Geometry: final body of the model. Coordinates: model frame, mm. A direction names the side the tool comes from. Give positions to 0.01 mm unless a question says otherwise; leave off trailing zeros. Write each loop counter-clockwise with the first axis right and the second up, starting at its lowest first coordinate (ties: lowest second). Pieces come first, ordered by that corner, then holes.
```python
from build123d import *

# Parameters (mm, degrees)
F0_W      = 69.85
F0_H      = 69.85
F1_DEPTH  = 1.5875
F2_W      = 69.85
F2_H      = 69.85
F2_W_2    = 66.675
F2_H_2    = 66.675
F3_DEPTH  = 42.8625
F4_W      = 60.325
F4_H      = 60.325
F4_W_2    = 57.15
F4_H_2    = 57.15
F5_DEPTH  = 74.6125
F6_W      = 57.15
F6_H      = 1.5875
F7_DEPTH  = 58.7375
F8_R      = 25.4
F9_DEPTH  = 74.6125
F10_R     = 26.9875
F10_R_2   = 25.4
F11_DEPTH = 76.2


with BuildPart() as f1:
    # F0 (on Top) → F1 (new body)
    with BuildSketch(Plane.XY):
        Rectangle(F0_W, F0_H)
    extrude(amount=F1_DEPTH)

    # F2 (on face) → F3 (join)
    with BuildSketch(Plane.XY.offset(1.5875)):
        Rectangle(F2_W, F2_H)
        Rectangle(F2_W_2, F2_H_2, mode=Mode.SUBTRACT)
    extrude(amount=F3_DEPTH)

    # F4 (on face) → F5 (join)
    with BuildSketch(Plane.XY.offset(1.5875)):
        Rectangle(F4_W, F4_H)
        Rectangle(F4_W_2, F4_H_2, mode=Mode.SUBTRACT)
    extrude(amount=F5_DEPTH)

    # F6 (on face) → F7 (join)
    with BuildSketch(Plane.YZ.offset(-28.575)):
        with Locations((0, 75.40625)):
            Rectangle(F6_W, F6_H)
    extrude(amount=F7_DEPTH)

    # F8 (on face) → F9 (cut)
    with BuildSketch(Plane.XY.offset(76.2)):
        Circle(F8_R)
    extrude(amount=-F9_DEPTH, mode=Mode.SUBTRACT)

    # F10 (on face) → F11 (join)
    with BuildSketch(Plane.XY.offset(76.2)):
        Circle(F10_R)
        Circle(F10_R_2, mode=Mode.SUBTRACT)
    extrude(amount=-F11_DEPTH)


solid = f1.part
```
Item 1: Pull-direction query (X, two-part tool) for faces 1 (the face through (-30.162, 0, 38)), 2 (the face through (0, -27, 76.2)); classes: +X half, -X half, draft (parallel to the pull), parting line (faces both ways), or undercut.
Found:
face 1: undercut
face 2: draft
Item 2: Line query: L1, parallel to Y at x = 0, z = 40 (1 decimal); L2, parallel to Y at x = 0, z = 53 (1 decimal); L3, parallel to X at y = 28.5, z = 52.5 (1 decimal). Output: solid intervals per line, ascending.
Found:
L1: y = -34.9 to -33.3, -30.2 to -28.6, -27 to -25.4, 25.4 to 27, 28.6 to 30.2, 33.3 to 34.9
L2: y = -30.2 to -28.6, -27 to -25.4, 25.4 to 27, 28.6 to 30.2
L3: x = -30.2 to -28.6, 28.6 to 30.2
Item 3: Section B-B, the plane x = 0. State how many separate pieces and enclosed holes the cut face has, plus the area to 3 significant figures.
Found:
separate pieces: 1
enclosed holes: 2
area: 726 mm2
Item 4: Section C-C, the plane z = 10. Return the cut outline in (x, y) (1 decimal), plus the area to 3 significant figures.
Found:
outline: (-34.9, -34.9) - (34.9, -34.9) - (34.9, 34.9) - (-34.9, 34.9) - close; (-30.2, -30.2) - (30.2, -30.2) - (30.2, 30.2) - (-30.2, 30.2) - close; circle Ø54 at (0, 0); hole (-33.3, -33.3) - (33.3, -33.3) - (33.3, 33.3) - (-33.3, 33.3) - close; hole (-28.6, -28.6) - (28.6, -28.6) - (28.6, 28.6) - (-28.6, 28.6) - close; hole circle Ø50.8 at (0, 0)
area: 1,070 mm2
Item 5: Pin query (flat end, axial travel): pin 1 Ø8 at (y, z) = (-16, 46.5) entering from +X (3 decimals); pin 2 Ø10 at (y, z) = (-3.5, 51) entering from +X; pin 3 Ø4 at (x, z) = (7.5, 56) entering from -Y; pin 4 Ø8 at (x, y) = (3, 7.5) entering from +Z. Return the tip coordinate at first contact, or that it passes through.
Found:
pin 1: stops at x = 34.925
pin 2: stops at x = 30.16
pin 3: stops at y = -30.16
pin 4: stops at z = 1.59
Item 6: Reachability of faces 3 (the face through (0, -28.575, 38)), 4 (the face through (-2.8, -33.5, 44.45)), 5 (the face through (0, 34.925, 22)) from +Z, -Z, +X, -X, +Y, -Y: full face, straight path, thin tool, end or side. Return the list, or none.
Found:
face 3: none
face 4: +Z
face 5: +Z, -Z, +X, -X, +Y
Item 7: Section A-A, the plane z = 53.5. Return the cut outline in (x, y) (1 decimal).
Found:
outline: (-30.2, -30.2) - (30.2, -30.2) - (30.2, 30.2) - (-30.2, 30.2) - close; circle Ø54 at (0, 0); hole (-28.6, -28.6) - (28.6, -28.6) - (28.6, 28.6) - (-28.6, 28.6) - close; hole circle Ø50.8 at (0, 0)
